from build123d import *

# Parameters (mm, degrees)
SKETCH1_R                    = 3.5
BOSS_EXTRUDE1_DEPTH          = 6.3
F_5_16_24_TAPPED_HOLE4_D     = 7.919999908
F_5_16_24_TAPPED_HOLE4_DEPTH = 12
F_5_16_24_TAPPED_HOLE4_TIP   = 2.379408024
SKETCH27_R                   = 6.421961615
SKETCH27_R_2                 = 3.97
BOSS_EXTRUDE2_DEPTH          = 1
FILLET2_R                    = 1
FILLET3_R                    = 0.5


with BuildPart() as part:
    # Sketch1 → Boss-Extrude1 (new body)
    with BuildSketch(Plane(origin=(0, 0, 0), x_dir=(1, 0, 0), z_dir=(0, 1, 0))):
        Polygon((3.70947548, -6.425), (7.418950959, 0), (3.70947548, 6.425), (-3.70947548, 6.425), (-7.418950959, 0), (-3.70947548, -6.425), align=None)
        with Locations(Location((0, 0, 0), (0, 0, 270))):
            Circle(SKETCH1_R, mode=Mode.SUBTRACT)
    extrude(amount=BOSS_EXTRUDE1_DEPTH)

    # Sketch3 → Cut-Revolve4 (revolve, cut)
    with BuildSketch(Plane.XY, mode=Mode.PRIVATE) as cut_revolve4_sk:
        Polygon((-6.421961615, 6.8), (-6.421961615, 6.3), (-7.421961615, 5.3), (-7.921961615, 5.3), (-7.921961615, 6.8), align=None)
        Polygon((-7.421961615, 1), (-6.421961615, 0), (-6.421961615, -0.5), (-7.921961615, -0.5), (-7.921961615, 1), align=None)
    revolve(cut_revolve4_sk.sketch.rotate(Axis((0, 0, 0), (0, 1, 0)), 120.000000074), axis=Axis((0, 0, 0), (0, 1, 0)), mode=Mode.SUBTRACT)

    # 5/16-24 Tapped Hole4
    with Locations(Plane.XZ):
        with Locations((0, 0)):
            Hole(F_5_16_24_TAPPED_HOLE4_D / 2, depth=F_5_16_24_TAPPED_HOLE4_DEPTH)
            with Locations((0, 0, -(F_5_16_24_TAPPED_HOLE4_DEPTH + F_5_16_24_TAPPED_HOLE4_TIP / 2))):  # 118° drill point
                Cone(0, F_5_16_24_TAPPED_HOLE4_D / 2, F_5_16_24_TAPPED_HOLE4_TIP, mode=Mode.SUBTRACT)

    # Sketch27 → Boss-Extrude2 (add)
    with BuildSketch(Plane.XZ):
        with Locations(Location((0, 0, 0), (0, 0, 270))):
            Circle(SKETCH27_R)
        with Locations(Location((0, 0, 0), (0, 0, 270))):
            Circle(SKETCH27_R_2, mode=Mode.SUBTRACT)
    extrude(amount=BOSS_EXTRUDE2_DEPTH)

    # Fillet2
    fillet2_edges = [part.edges().sort_by_distance(p)[0] for p in [
        (0, -1, 6.421961615),
    ]]
    fillet(fillet2_edges, radius=FILLET2_R - 0.0001)  # a hair under: the kernel refuses the full size

    # Fillet3
    fillet3_edges = [part.edges().sort_by_distance(p)[0] for p in [
        (0, -1, 3.97),
    ]]
    fillet(fillet3_edges, radius=FILLET3_R)


solid = part.part
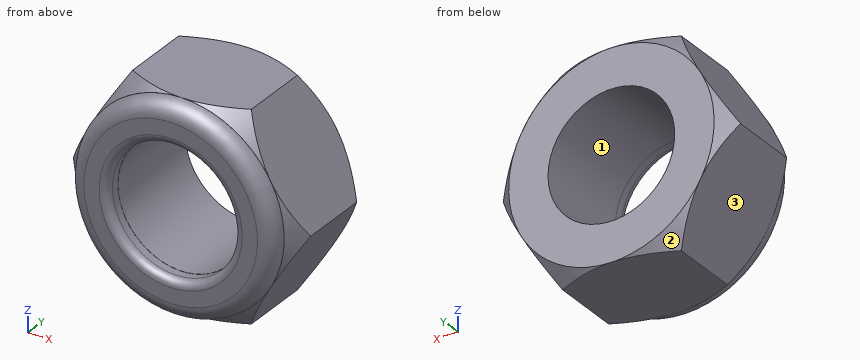
Model file for the job. Use its own axes, mm. Face numbers are marked on the shaded views. Round coordinates to 2 decimals unless told otherwise and drop trailing zeros. Order: outer loops, then holes, each group sorted by start corner. A loop starts at its lowest first (then second) coordinate and runs counter-clockwise, first axis right, second up.
(1) Pin check, flat tips, straight feed: pin 1 (2 mm diameter, centred on x = -5, y = 5.5, fed in from -Z); pin 2 (7 mm diameter, centred on x = 0, z = 0, fed in from -Y); pin 3 (3 mm diameter, centred on y = 3.5, z = -2.5, fed in from -X). Stop position of each tip, or through.
(2) Drill centre lines: line 1 (Z direction, x = 0, y = 3.25) (3 decimals); line 2 (X direction, y = 2, z = 1.5); line 3 (X direction, y = 3.25, z = -2.75). Where is each one in solid material? Low to high.
(3) Band-saw the part on C-C (y = 0.25). List the corners of the cut face in (x, z) (3 decimals), then the cut area to 3 significant figures.
(4) Pull direction X, two halves, no side cores. Call the marked faces 1, 2 and 3: released by +X, released by -X, zero draft, split by the parting line, or undercut.
(5) Band-saw the part on B-B (y = 1.75). List the corners of the cut face in (x, z) (3 decimals), then the cut area to 3 significant figures.
Verdict:
1. pin 1: stops at z = -5.92
1. pin 2: passes through
1. pin 3: stops at x = -6.84
2. line 1: z = -6.425 to -3.96, 3.96 to 6.425
2. line 2: x = -6.55 to -3.66, 3.66 to 6.55
2. line 3: x = -5.83 to -2.85, 2.85 to 5.83
3. outline: (-6.463, -1.655) - (-4.665, -4.77) arc R6.672 ccw to (-1.798, -6.425) - (1.798, -6.425) arc R6.672 ccw to (4.665, -4.77) - (6.463, -1.655) arc R6.672 ccw to (6.463, 1.655) - (4.665, 4.77) arc R6.672 ccw to (1.798, 6.425) - (-1.798, 6.425) arc R6.672 ccw to (-4.665, 4.77) - (-6.463, 1.655) arc R6.672 ccw to start; hole circle Ø7.92 at (0, 0)
3. area: 87.0 mm2
4. face 1: undercut
4. face 2: split by the parting line
4. face 3: released by -X
5. outline: (-7.419, 0) - (-3.709, -6.425) - (3.709, -6.425) - (7.419, 0) - (3.709, 6.425) - (-3.709, 6.425) - close; hole circle Ø7.92 at (0, 0)
5. area: 93.7 mm2
